Part model, mm, in its own coordinate system. Face numbers are marked on the shaded views. A direction names the side the tool comes from. Coordinates: 2 decimals unless noted, no trailing zeros. Order: outer loops, then holes, each group sorted by start corner. A loop starts at its lowest first (then second) coordinate and runs counter-clockwise, first axis right, second up.
Autodesk Fusion 360 part; units mm, degrees
sketch "Esquisse1" plane through (0, 0, 0) normal (0, 0, 1) x (1, 0, 0)
  line L0 (21, -7.5) -> (-21, -7.5)
  line L1 (-21, -7.5) -> (-21, 7.5)
  line L2 (21, 7.5) -> (21, -7.5)
  line L3 (21, -7.5) -> (-21, 7.5) construction
  line L4 (-21, -7.5) -> (21, 7.5) construction
  circle A0 centre (5, -4.5) radius 1.75
  circle A1 centre (-9, -4.5) radius 1.75
  line L5 (-9, -4.5) -> (5, -4.5) construction
  line L6 (-9, -4.5) -> (-9, -7.5) construction
  line L7 (-9, -4.5) -> (-21, -4.5) construction
  line L8 (5, -4.5) -> (21, -4.5) construction
  line L9 (-21, 7.5) -> (21, 7.5)
  line L10 (-21, 7.5) -> (-4, 7.5)
  line L11 (-4, 9) -> (-4, 5.805) construction
  dimension "d1" = 42
  dimension "d2" = 15
  dimension "d3" = 3.5
  dimension "d4" = 3.5
  dimension "d6" = 3
  dimension "d42" = 12
  dimension "d43" = 14
  dimension "d44" = 16
  dimension "d64" = 17
extrude "Extrusion1" add sketch "Esquisse1" along normal blind 4
sketch "Esquisse6" plane through (0, 0, 0) normal (0, 0, 1) x (1, 0, 0)
  line L0 (21, 7.5) -> (23, 7.5)
  line L1 (23, 7.5) -> (23, -27.5)
  line L2 (23, -27.5) -> (21, -27.5)
  line L3 (21, -27.5) -> (21, 7.5)
  dimension "d45" = 2
  dimension "d46" = 35
extrude "Extrusion6" add sketch "Esquisse6" along normal blind 15
sketch "Esquisse7" plane through (0, 0, 4) normal (0, 0, 1) x (-1, 0, 0)
  circle A0 centre (-5, 4.5) radius 1.75
  circle A1 centre (9, 4.5) radius 1.75
  line L0 (21, -7.5) -> (21, 7.5)
  line L1 (21, 7.5) -> (-21, 7.5)
  line L2 (-21, 7.5) -> (-21, -7.5)
  line L3 (-21, -7.5) -> (21, -7.5)
  line L4 (-21, 4.0051) -> (-21, 7.5)
  line L5 (-21, 7.5) -> (-5, 7.5)
  line L6 (-8.9589, 4.0051) -> (-21, 4.0051)
  arc A2 (-6, 7.5) -> (-8.9589, 4.0051) centre (-6, 4.5) ccw
  dimension "d70" = 6
extrude "Extrusion7" cut sketch "Esquisse7" against normal blind 4 contours L1 L2 L4 L5 L6 A2
chamfer "Chanfrein3" distance 1.5 angle 45 1 edges at (-21, -7.5, 2)
fillet "Congé10" radius 2 1 edges at (21, 1.7475, 4)
fillet "Congé11" radius 2 1 edges at (21, -4.0051, 3)
fillet "Congé12" radius 2 1 edges at (22, 7.5, 15)
fillet "Congé13" radius 2 1 edges at (22, -27.5, 15)
hole "Perçage1" at (-3.9685, 7.9961, 4) direction (0, 0, -1) diameter 8 end through all
chamfer "Chanfrein5" distance 1.5 angle 45 1 edges at (-21, 7.5, 2)
fillet "Congé14" radius 2 1 edges at (8.9589, -4.0051, 2)
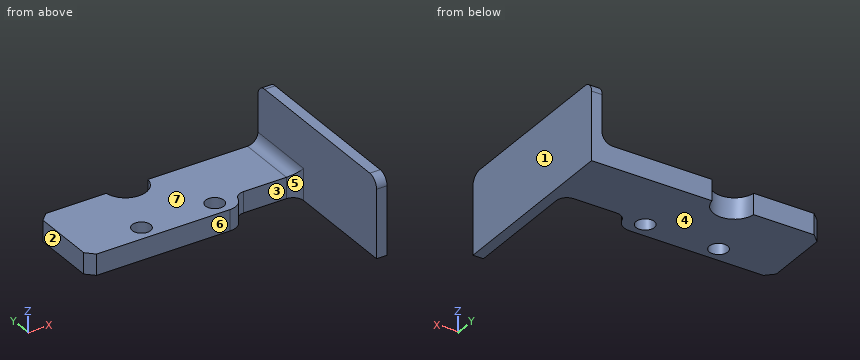
Q1. Mould opens along X. For the marked faces 1, 2 and 3 say: pulls with the +X half, pulls with the -X half, needs draft (parallel to the pull), parting line crosses it, or undercut.
Results list:
face 1: pulls with the +X half
face 2: pulls with the -X half
face 3: undercut
Q2. Cut at A-A on z = 2.25. Write the cut outline in (x, y).
Results list:
outline: (-21, -6) - (-19.5, -7.5) - (6, -7.5) arc R3 ccw to (8.86, -5.4) arc R2 cw to (10.77, -4.01) - (19, -4.01) arc R2 cw to (21, -6.01) - (21, -27.5) - (23, -27.5) - (23, 7.5) - (0, 7.5) arc R4 cw to (-7.94, 7.5) - (-19.5, 7.5) - (-21, 6) - close; hole circle Ø3.5 at (-9, -4.5); hole circle Ø3.5 at (5, -4.5)
Q3. Pin check, flat tips, straight feed: pin 1 Ø1 at (y, z) = (-23, 6.5) entering from -X; pin 2 Ø4.5 at (x, z) = (15.5, 3) entering from -Y; pin 3 Ø12 at (x, y) = (0.5, -3.5) entering from +Z; pin 4 Ø3 at (x, y) = (5, -4.5) entering from -Z. Stop position of each tip, or through.
Results list:
pin 1: stops at x = 21
pin 2: stops at y = -4.01
pin 3: stops at z = 4
pin 4: passes through
Q4. Cut at C-C on y = -4.5. Write the cut outline in (x, z), and give its area (3 significant figures).
Results list:
outline: (-21, 0) - (-10.75, 0) - (-10.75, 4) - (-21, 4) - close; (-7.25, 0) - (3.25, 0) - (3.25, 4) - (-7.25, 4) - close; (6.75, 0) - (9.45, 0) - (9.45, 4) - (6.75, 4) - close; (20.32, 0) - (23, 0) - (23, 15) - (21, 15) - (21, 6) arc R2 cw to (20.32, 4.49) - close
area: 127 mm2
Q5. Cut at B-B on x = 5. Write the cut outline in (y, z), and give its area (3 significant figures).
Results list:
outline: (-7.5, 0) - (-6.25, 0) - (-6.25, 4) - (-7.5, 4) - close; (-2.75, 0) - (7.5, 0) - (7.5, 4) - (-2.75, 4) - close
area: 46.0 mm2
Q6. Which spindle directions (+Z, -Z, +X, -X, +Y, -Y) get a long thin tool onto all of the face, cutting with end or side? Do the marked faces 4, 5, 6 and 7. Say none if no direction does.
Results list:
face 4: -Z, +X, -X, +Y, -Y
face 5: +Z, -Z, -Y
face 6: +Z, -Z, -X, -Y
face 7: +Z, -X, +Y, -Y
Q7. Cut at D-D on z = 12. Write the cut outline in (x, y), and give its area (3 significant figures).
Results list:
outline: (21, -27.5) - (23, -27.5) - (23, 7.5) - (21, 7.5) - close
area: 70.0 mm2
Q8. Wall check: line 1 along Y through (x, z) = (5, 2.3); line 2 along X through (y, z) = (-19, 2.5); line 3 along Z through (x, y) = (10, -3). Give the ranges that are in metal, low to high.
Results list:
line 1: y = -7.5 to -6.25, -2.75 to 7.5
line 2: x = 21 to 23
line 3: z = 0 to 4
